Verification items for the finished model (mm, model axes). A direction names the side the tool comes from. Round coordinates to 2 decimals unless told otherwise and drop trailing zeros. Write each loop counter-clockwise with the first axis right and the second up, starting at its lowest first coordinate (ties: lowest second). Pieces come first, ordered by that corner, then holes. Notation, with made-up numbers: M 46.5,-38 L 89.5,-38 A18 cw 89.5,-24 Z; hole C 5,88 d3. An arc over 180 degrees is marked long. One line per question, with ' | ' between items. Start each with the question number.
Q1. Gauge pin test, flat ends, axial feed: pin 1 (0.9 mm diameter, centred on x = -31.5, y = -1.5, fed in from +Z); pin 2 (2.5 mm diameter, centred on x = 29.5, y = -8, fed in from +Z); pin 3 (1.8 mm diameter, centred on y = -4, z = -2, fed in from +X) (3 decimals). Record the tip position at first contact, or that the pin passes through.
Q2. Tool access check on faces 1 (the face through (31.35, -4, 25)), 2 (the face through (47, -5, 3.417)), 3 (the face through (-24.5, -5, -28)), 4 (the face through (46.225, -5, -2)). Record the directions out of +Z, -Z, +X, -X, +Y, -Y that give a thin tool (end or side, any length) a straight path to the whole face; none if there is none.
Q3. Cross-section at C-C (x = -38.5). Record the boundary of the cut face in (y, z).
Q4. Cross-section at A-A (z = -13). Record the boundary of the cut face in (x, y).
Q5. Cross-section at B-B (x = -12.5). Record the boundary of the cut face in (y, z).
Q6. Thickness scan on line 1 along Z through (x, y) = (-26.5, -9); line 2 along X through (y, z) = (1.55, 13); line 3 along X through (y, z) = (1.35, -13). Record the ranges inside material, lowest first. Write a range as from..to.
Q7. Release check for a two-part mould opening along Z. For faces 5 (the face through (30, -9.8, -27)), 6 (the face through (30.43, -5.64, 29.24)), 7 (the face through (-27, -5, 26.5)) record: released by +Z, released by -Z, zero draft, split by the parting line, or undercut.
Q8. Cross-section at D-D (y = -5.5). State how many separate pieces and enclosed holes the cut face has, then the cut area to 3 significant figures.
from build123d import *

# Parameters (mm, degrees)
BOSS_EXTRUDE1_DEPTH     = 2.5
FILLET1_R               = 5
BOSS_EXTRUDE2_DEPTH     = 9.8
CUT_EXTRUDE1_DEPTH      = 9.8
CUT_EXTRUDE2_DEPTH      = 89.657557489
BOSS_EXTRUDE3_DEPTH     = 11.7
MIRROR4_COPY_1_DEPTH    = 11.7
CUT_EXTRUDE3_DEPTH      = 61.401076149
CUT_EXTRUDE3_DEPTH_BACK = 61.401076149
SKETCH7_R               = 10.4
SKETCH7_R_2             = 5.75


with BuildPart() as part:
    # Sketch1 → Boss-Extrude1 (new body)
    with BuildSketch(Plane(origin=(0, 0, 0), x_dir=(1, 0, 0), z_dir=(0, 1, 0))):
        with BuildLine():
            Line((-46.5, 30), (46.5, 30))
            ThreePointArc((46.5, 30), (50.035533906, 28.535533906), (51.5, 25))
            Line((51.5, 25), (51.5, -25))
            ThreePointArc((51.5, -25), (50.035533906, -28.535533906), (46.5, -30))
            Line((46.5, -30), (-46.5, -30))
            ThreePointArc((-46.5, -30), (-50.035533906, -28.535533906), (-51.5, -25))
            Line((-51.5, -25), (-51.5, 25))
            ThreePointArc((-51.5, 25), (-50.035533906, 28.535533906), (-46.5, 30))
        make_face()
    extrude(amount=BOSS_EXTRUDE1_DEPTH)

    # Fillet1
    # the kernel refuses this fillet: 5 mm, written as the material it takes off along each edge
    with BuildSketch(Plane(origin=(-46.5, 2.5, -25), x_dir=(-1, 0, 0), z_dir=(0, 0, 1))) as fillet1_piece_1:
        with BuildLine():
            CenterArc((0.669872981, 5), FILLET1_R, 270, 60)
            Line((0.669872981, 0), (0.669872981, -0.1))
            Line((0.669872981, -0.1), (5, -0.1))
            Line((5, -0.1), (5.1, 0))
            ThreePointArc((5.1, 0), (5.1, 1.25), (5.08660254, 2.45))
            Line((5.08660254, 2.45), (5, 2.5))
        make_face()
    revolve(axis=Axis((-46.5, 2.5, -25), (0, -1, 0)), revolution_arc=90, mode=Mode.SUBTRACT)
    with BuildSketch(Plane(origin=(-46.5, 2.5, -30), x_dir=(0, -1, 0), z_dir=(1, 0, 0)), Plane(origin=(46.5, 2.5, 30), x_dir=(0, -1, 0), z_dir=(-1, 0, 0))) as fillet1_piece_2:
        with BuildLine():
            CenterArc((5, -4.330127019), FILLET1_R, 120, 60)
            Line((0, -4.330127019), (-0.1, -4.330127019))
            Line((-0.1, -4.330127019), (-0.1, 0))
            Line((-0.1, 0), (0, 0.1))
            ThreePointArc((0, 0.1), (1.25, 0.1), (2.45, 0.08660254))
            Line((2.45, 0.08660254), (2.5, 0))
        make_face()
    extrude(amount=93, mode=Mode.SUBTRACT)
    with BuildSketch(Plane(origin=(46.5, 2.5, -25), x_dir=(0, 0, -1), z_dir=(-1, 0, 0))) as fillet1_piece_3:
        with BuildLine():
            CenterArc((0.669872981, 5), FILLET1_R, 270, 60)
            Line((0.669872981, 0), (0.669872981, -0.1))
            Line((0.669872981, -0.1), (5, -0.1))
            Line((5, -0.1), (5.1, 0))
            ThreePointArc((5.1, 0), (5.1, 1.25), (5.08660254, 2.45))
            Line((5.08660254, 2.45), (5, 2.5))
        make_face()
    revolve(axis=Axis((46.5, 2.5, -25), (0, -1, 0)), revolution_arc=90, mode=Mode.SUBTRACT)
    with BuildSketch(Plane(origin=(51.5, 2.5, -25), x_dir=(0, -1, 0), z_dir=(0, 0, 1)), Plane(origin=(-51.5, 2.5, 25), x_dir=(0, -1, 0), z_dir=(0, 0, -1))) as fillet1_piece_4:
        with BuildLine():
            CenterArc((5, -4.330127019), FILLET1_R, 120, 60)
            Line((0, -4.330127019), (-0.1, -4.330127019))
            Line((-0.1, -4.330127019), (-0.1, 0))
            Line((-0.1, 0), (0, 0.1))
            ThreePointArc((0, 0.1), (1.25, 0.1), (2.45, 0.08660254))
            Line((2.45, 0.08660254), (2.5, 0))
        make_face()
    extrude(amount=50, mode=Mode.SUBTRACT)
    with BuildSketch(Plane(origin=(46.5, 2.5, 25), x_dir=(1, 0, 0), z_dir=(0, 0, -1))) as fillet1_piece_5:
        with BuildLine():
            CenterArc((0.669872981, 5), FILLET1_R, 270, 60)
            Line((0.669872981, 0), (0.669872981, -0.1))
            Line((0.669872981, -0.1), (5, -0.1))
            Line((5, -0.1), (5.1, 0))
            ThreePointArc((5.1, 0), (5.1, 1.25), (5.08660254, 2.45))
            Line((5.08660254, 2.45), (5, 2.5))
        make_face()
    revolve(axis=Axis((46.5, 2.5, 25), (0, -1, 0)), revolution_arc=90, mode=Mode.SUBTRACT)
    with BuildSketch(Plane(origin=(-46.5, 2.5, 25), x_dir=(0, 0, 1), z_dir=(1, 0, 0))) as fillet1_piece_6:
        with BuildLine():
            CenterArc((0.669872981, 5), FILLET1_R, 270, 60)
            Line((0.669872981, 0), (0.669872981, -0.1))
            Line((0.669872981, -0.1), (5, -0.1))
            Line((5, -0.1), (5.1, 0))
            ThreePointArc((5.1, 0), (5.1, 1.25), (5.08660254, 2.45))
            Line((5.08660254, 2.45), (5, 2.5))
        make_face()
    revolve(axis=Axis((-46.5, 2.5, 25), (0, -1, 0)), revolution_arc=90, mode=Mode.SUBTRACT)

    # Sketch2 → Boss-Extrude2 (add)
    with BuildSketch(Plane.XZ):
        Polygon((-36.2, 28.5), (-24.5, 28.5), (-24.5, 26.5), (-29.35, 26.5), (-29.35, 20.5), (-31.35, 20.5), (-31.35, 26.5), (-36.2, 26.5), align=None)
        Polygon((48.225, -3.282847821), (46.225, -3.282847821), (46.225, -0.999790058), (40.225, -0.999790058), (40.225, 1), (46.225, 1), (46.225, 3.417152179), (48.225, 3.417152179), align=None)
        Polygon((24.5, 28.5), (36.2, 28.5), (36.2, 26.5), (31.35, 26.5), (31.35, 20.5), (29.35, 20.5), (29.35, 26.5), (24.5, 26.5), align=None)
        Polygon((24.5, -26.5), (29.35, -26.5), (29.35, -20.5), (31.35, -20.5), (31.35, -26.5), (36.2, -26.5), (36.2, -28.5), (24.5, -28.5), align=None)
        Polygon((-36.2, -28.5), (-24.5, -28.5), (-24.5, -26.5), (-29.35, -26.5), (-29.35, -20.5), (-31.35, -20.5), (-31.35, -26.5), (-36.2, -26.5), align=None)
        Polygon((-48.225, 3.417152179), (-46.225, 3.417152179), (-46.225, 1), (-40.225, 1), (-40.225, -0.999790058), (-46.225, -0.999790058), (-46.225, -3.282847821), (-48.225, -3.282847821), align=None)
    extrude(amount=BOSS_EXTRUDE2_DEPTH)

    # Sketch4 → Cut-Extrude1 (cut)
    with BuildSketch(Plane(origin=(0, 0, -0.999790058), x_dir=(-1, 0, 0), z_dir=(0, 0, -1))):
        Polygon((40.225, 0), (46.225, -9.8), (40.225, -9.8), align=None)
    cut_extrude1 = extrude(amount=-CUT_EXTRUDE1_DEPTH, mode=Mode.SUBTRACT)

    # Mirror1: Cut-Extrude1 across plane
    add(cut_extrude1.mirror(Plane(origin=(0, 0, 0), x_dir=(0, 0, 1), z_dir=(1, 0, 0))), mode=Mode.SUBTRACT)

    # Sketch5 → Cut-Extrude2 (cut, through all)
    with BuildSketch(Plane.ZY.offset(31.35)):
        Polygon((-26.5, -9.8), (-20.5, 0), (-20.5, -9.8), align=None)
    cut_extrude2 = extrude(amount=-CUT_EXTRUDE2_DEPTH, mode=Mode.SUBTRACT)

    # Mirror2: Cut-Extrude2 across plane
    add(cut_extrude2.mirror(Plane.XY), mode=Mode.SUBTRACT)

    # Sketch6 → Boss-Extrude3 (add)
    with BuildSketch(Plane(origin=(36.2, 0, 0), x_dir=(0, 0, -1), z_dir=(1, 0, 0))):
        Polygon((-28.5, -3), (-28.5, -7.5), (-30, -3.726144837), align=None)
    boss_extrude3 = extrude(amount=-BOSS_EXTRUDE3_DEPTH)

    # Mirror3: Boss-Extrude3 across plane
    add(boss_extrude3.mirror(Plane(origin=(0, 0, 0), x_dir=(0, 0, 1), z_dir=(1, 0, 0))))

    # Mirror4: Boss-Extrude3 across plane
    add(boss_extrude3.mirror(Plane.XY))

    # Mirror4 copy 1 sketch → Mirror4 copy 1 (add)
    with BuildSketch(Plane.ZY.offset(36.2)):
        Polygon((-28.5, -3), (-28.5, -7.5), (-30, -3.726144837), align=None)
    extrude(amount=-MIRROR4_COPY_1_DEPTH)

    # Sketch7 → Cut-Extrude3 (cut, two sides: drawn at the far end of the back side and taken through both)
    with BuildSketch(Plane.XZ.offset(-CUT_EXTRUDE3_DEPTH_BACK)):
        with Locations(Location((-37.5, 13, 0), (0, 0, 201.597043682))):
            Circle(SKETCH7_R)
        with Locations(Location((-12.5, 13, 0), (0, 0, 270))):
            Circle(SKETCH7_R)
        with Locations(Location((-36.5, -13, 0), (0, 0, 270))):
            Circle(SKETCH7_R_2)
        with Locations(Location((12.5, 13, 0), (0, 0, 270))):
            Circle(SKETCH7_R)
        with Locations(Location((37.5, 13, 0), (0, 0, 338.402956318))):
            Circle(SKETCH7_R)
        with Locations(Location((-12.5, -13, 0), (0, 0, 270))):
            Circle(SKETCH7_R_2)
        with Locations(Location((12.5, -13, 0), (0, 0, 90))):
            Circle(SKETCH7_R_2)
        with Locations(Location((36.5, -13, 0), (0, 0, 90))):
            Circle(SKETCH7_R_2)
    extrude(amount=CUT_EXTRUDE3_DEPTH + CUT_EXTRUDE3_DEPTH_BACK, mode=Mode.SUBTRACT)


solid = part.part
Determined:
1) pin 1: stops at z = 28.5 | pin 2: stops at z = 28.8 | pin 3: stops at x = 48.225
2) face 1: +X, -Y | face 2: +Z, +X, -X, -Y | face 3: +Z, -Z, -Y | face 4: -Z, -Y
3) outline: M 0,-30 A5 ccw 2.5,-25.67 L 2.5,-18.39 L 0,-18.39 Z; M 0,-7.61 L 2.5,-7.61 L 2.5,2.65 L 0,2.65 Z; M 0,23.35 L 2.5,23.35 L 2.5,25.67 A5 ccw 0,30 Z
4) outline: M -51.5,0 L -42.25,0 L -42.25,2.5 L -47.17,2.5 A5 ccw Z; M -30.75,0 L -18.25,0 L -18.25,2.5 L -30.75,2.5 Z; M -6.75,0 L 6.75,0 L 6.75,2.5 L -6.75,2.5 Z; M 18.25,0 L 30.75,0 L 30.75,2.5 L 18.25,2.5 Z; M 42.25,0 L 51.5,0 A5 ccw 47.17,2.5 L 42.25,2.5 Z
5) outline: M 0,-30 A5 ccw 2.5,-25.67 L 2.5,-18.75 L 0,-18.75 Z; M 0,-7.25 L 2.5,-7.25 L 2.5,2.6 L 0,2.6 Z; M 0,23.4 L 2.5,23.4 L 2.5,25.67 A5 ccw 0,30 Z
6) line 1: z = -28.5..-26.5, 26.5..28.5 | line 2: x = -50.1..-47.9, -27.1..-22.9, -2.1..2.1, 22.9..27.1, 47.9..50.1 | line 3: x = -50.36..-42.25, -30.75..-18.25, -6.75..6.75, 18.25..30.75, 42.25..50.36
7) face 5: zero draft | face 6: released by +Z | face 7: undercut
8) separate pieces: 6 | enclosed holes: 0 | area: 189 mm²
